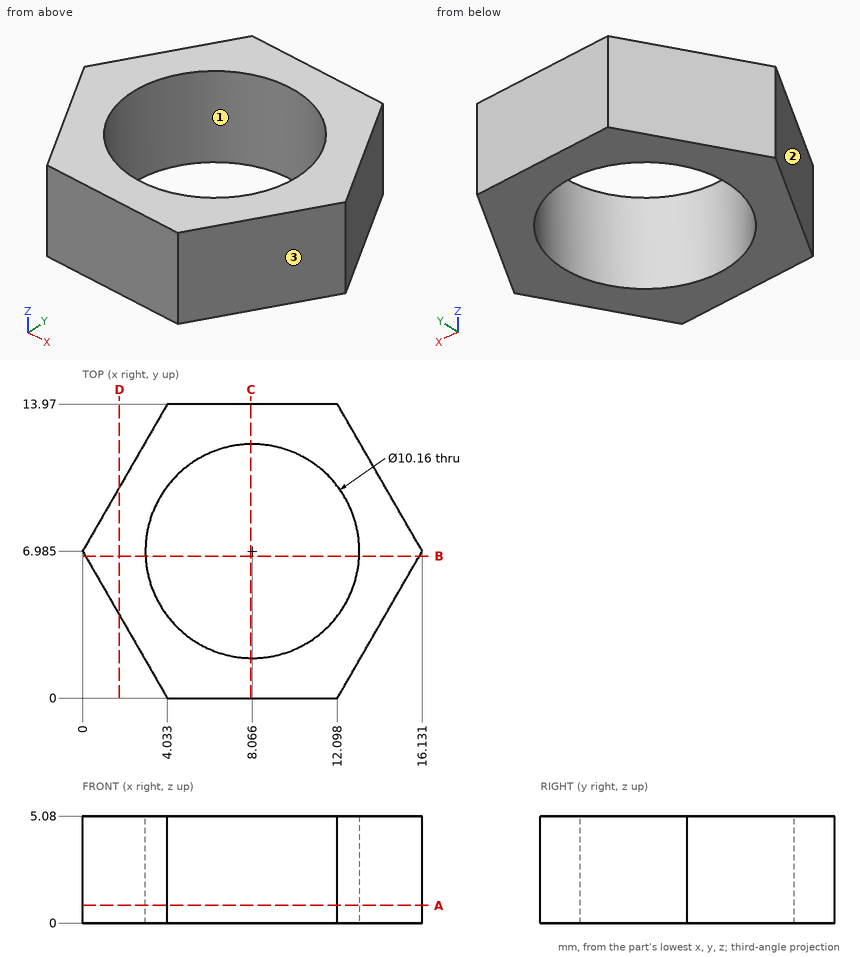
Design review of the part shown in the three views and the two pictorial views. Dimensions are in mm from the part's minimum x, y and z. Coordinates: 2 decimals unless noted, no trailing zeros. Write each loop counter-clockwise with the first axis right and the second up, starting at its lowest first coordinate (ties: lowest second). Pieces come first, ordered by that corner, then holes.
1) We need section B-B on y = 6.75. State the section outline as (x, z) points (1 decimal).
2) We need section D-D on x = 1.75. State the section outline as (y, z) points.
3) Clearance check with flat-ended pins moving along their axes: pin 1 Ø1 at (y, z) = (12, 4) entering from -X; pin 2 Ø1 at (y, z) = (10, 3) entering from +X; pin 3 Ø1.5 at (y, z) = (9.5, 2.5) entering from +X; pin 4 Ø5 at (x, y) = (11, 3) entering from -Z. State where each tip first meets the part, or that it passes through.
4) We need section C-C on x = 8. State the section outline as (y, z) points (1 decimal).
5) The part is to be moulded in two halves that separate along X. For the marked faces 1, 2 and 3, say which applies: pulls with the +X half, pulls with the -X half, needs draft (parallel to the pull), parting line crosses it, or undercut.
6) We need section A-A on z = 0.85. State the section outline as (x, y) points (1 decimal).
7) To check wall thickness, follow probe 1 along X at (y, z) = (4.75, 3.95) (1 decimal); probe 2 along X at (y, z) = (6.5, 2.55); probe 3 along Y at (x, z) = (10, 3.35). State the ranges of each line that lie inside material, in increasing order.
Answer list:
1. outline: (0.1, 0) - (3, 0) - (3, 5.1) - (0.1, 5.1) - close; (13.1, 0) - (16, 0) - (16, 5.1) - (13.1, 5.1) - close
2. outline: (3.95, 0) - (10.02, 0) - (10.02, 5.08) - (3.95, 5.08) - close
3. pin 1: stops at x = 2.61
3. pin 2: stops at x = 14.68
3. pin 3: stops at x = 15.11
3. pin 4: stops at z = 0
4. outline: (0, 0) - (1.9, 0) - (1.9, 5.1) - (0, 5.1) - close; (12.1, 0) - (14, 0) - (14, 5.1) - (12.1, 5.1) - close
5. face 1: undercut
5. face 2: pulls with the -X half
5. face 3: pulls with the +X half
6. outline: (0, 7) - (4, 0) - (12.1, 0) - (16.1, 7) - (12.1, 14) - (4, 14) - close; hole circle Ø10.2 at (8.1, 7)
7. probe 1: x = 1.3 to 3.5, 12.6 to 14.8
7. probe 2: x = 0.28 to 3.01, 13.12 to 15.85
7. probe 3: y = 0 to 2.29, 11.68 to 13.97
